Geometry: final body of the model. Coordinates: model frame, mm. Face numbers are marked on the shaded views. A direction names the side the tool comes from. Round coordinates to 2 decimals unless told otherwise and drop trailing zeros. Write each loop counter-clockwise with the first axis right and the second up, starting at its lowest first coordinate (ties: lowest second). Pieces come first, ordered by that corner, then holes. Notation, with made-up numbers: (-11, 60.5) - (30, 60.5) arc R11 cw to (30, 68.5) - close; hole circle Ø8 at (-25.75, 55). An arc over 180 degrees is marked (long way). Write each question's results on one line, items separated by ' | '.
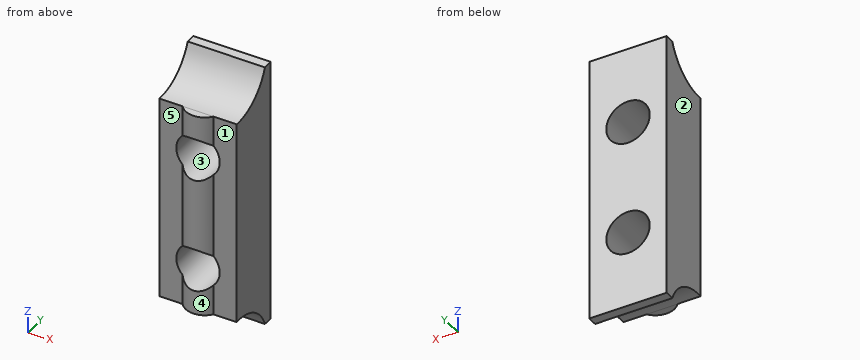
Autodesk Inventor part; units mm, degrees
ref_plane "Work Plane1" through (0, 0, 3.2) normal (0, 0, -1) x (-1, 0, 0)
ref_plane "YZ Plane" through (0, 0, 0) normal (1, 0, 0) x (0, 1, 0)
ref_plane "XZ Plane" through (0, 0, 0) normal (0, 1, 0) x (-1, 0, 0)
sketch "Sketch1" plane through (0, 0, 0) normal (0, 0, 1) x (1, 0, 0)
  line L0 (0, 0) -> (8, 0)
  line L1 (8, 0) -> (8, 6)
  line L2 (8, 6) -> (0, 6)
  line L3 (0, 6) -> (0, 0)
  dimension "d0" = 8
  dimension "d1" = 6
extrude "Extrusion1" add sketch "Sketch1" along normal blind 27.9
sketch "Sketch3" plane through (8, 0, 0) normal (1, 0, 0) x (0, 0, -1)
  line L0 (0, 0) -> (0, 6)
  line L1 (-27.9, 0) -> (-27.9, 6)
  line L2 (0, 0) -> (-27.9, 0)
  arc A0 (-24.7, 0) -> (-27.9, 5) centre (-29.689, 0.331) ccw
  arc A1 (0, 5) -> (-3.2, 0) centre (1.789, 0.331) ccw
  dimension "d14" = 5
  dimension "d15" = 3.2
  dimension "d16" = 1
extrude "Extrusion2" cut sketch "Sketch3" against normal up to next
ref_plane "Work Plane1" through (0, 0, 3.2) normal (0, 0, -1) x (-1, 0, 0)
sketch "Sketch4" plane through (0, 0, 3.2) normal (0, 0, -1) x (-1, 0, 0)
  line L0 (0, 0) -> (-8, 0)
  line L1 (-8, 0) -> (0, 0)
  arc A0 (-5.6, 0) -> (-2.4, 0) centre (-4, 1.2) ccw
  line L2 (-8, 0) -> (-8, 5)
  line L3 (-5.6, 0) -> (-2.4, 0)
  dimension "d20" = 2
  dimension "d21" = 4
  dimension "d22" = 1.2
extrude "Extrusion3" add sketch "Sketch4" against normal blind 21.5
sketch "Sketch2" plane through (0, 6, 0) normal (0, 1, 0) x (1, 0, 0)
  line L0 (8, -27.9) -> (0, -27.9)
  line L1 (8, 0) -> (8, -27.9)
  point P0 (4, -7.95)
  point P1 (4, -19.95)
  dimension "d4" = 12
  dimension "d5" = 7.95
  dimension "d6" = 4
hole "Hole1" at (4, 6, 7.95) at (4, 6, 19.95) direction (0, -1, 0) diameter 4.5 end through all
properties part number "Infill3DSpringHandle" material "ABS Plastic"
Q1. Ray query, line 1 along X through (y, z) = (3.5, 7.95); line 2 along Z through (x, y) = (4, 2.5); line 3 along Z through (x, y) = (3.75, 0). Return the intervals inside material, ascending.
Answer block:
line 1: 0 to 1.75, 6.25 to 8 | line 2: 2.72 to 5.7, 10.2 to 17.7, 22.2 to 25.18 | line 3: 3.2 to 5.71, 10.19 to 17.71, 22.19 to 24.7
Q2. Section query A-A, the plane x = 4. Return loops of the section in (y, z).
Answer block:
outline: (-0.8, 3.2) - (0, 3.2) arc R5 cw to (5, 0) - (6, 0) - (6, 5.7) - (-0.8, 5.7) - close; (-0.8, 10.2) - (6, 10.2) - (6, 17.7) - (-0.8, 17.7) - close; (-0.8, 22.2) - (6, 22.2) - (6, 27.9) - (5, 27.9) arc R5 cw to (0, 24.7) - (-0.8, 24.7) - close
Q3. Pin query (flat end, axial travel): pin 1 (2 mm diameter, centred on x = 3, y = 4.5, fed in from +Z); pin 2 (0.9 mm diameter, centred on x = 3.5, y = -0.5, fed in from -Z); pin 3 (2.5 mm diameter, centred on x = 7.5, z = 12, fed in from -Y); pin 4 (1.5 mm diameter, centred on x = 5, z = 23, fed in from -Y). Return the tip coordinate at first contact, or that it passes through.
Answer block:
pin 1: z = 27.9 | pin 2: z = 3.2 | pin 3: y = 0 | pin 4: y = -0.78
Q4. Access query for the marked faces 1 and 2. Directions: +Z, -Z, +X, -X, +Y, -Y. A direction counts if a zero-diameter tool reaches every point of the face in a straight line with its end or side. Return the directions, or none.
Answer block:
face 1: +Z, -Z, +X, -Y | face 2: +Z, -Z, -X, +Y, -Y
Q5. Section query B-B, the plane z = 19.95. Return loops of the section in (x, y), plus the area to 3 significant figures.
Answer block:
outline: (0, 0) - (1.75, 0) - (1.75, 6) - (0, 6) - close; (6.25, 0) - (8, 0) - (8, 6) - (6.25, 6) - close | area: 21.0 mm2
Q6. Section query D-D, the plane z = 13. Return loops of the section in (x, y), plus the area to 3 significant figures.
Answer block:
outline: (0, 0) - (2.4, 0) arc R2 ccw to (5.6, 0) - (8, 0) - (8, 6) - (0, 6) - close | area: 49.8 mm2
Q7. Section query C-C, the plane y = 1.5. Return loops of the section in (x, z).
Answer block:
outline: (0, 3.07) - (8, 3.07) - (8, 24.83) - (0, 24.83) - close; hole circle Ø4.5 at (4, 7.95); hole circle Ø4.5 at (4, 19.95)
Q8. Mould query, pull axis X, two halves, no side actions, for the marked faces 3, 4 and 5. Classes: pulls with the +X half, pulls with the -X half, needs draft (parallel to the pull), parting line crosses it, or undercut.
Answer block:
face 3: undercut | face 4: parting line crosses it | face 5: needs draft
